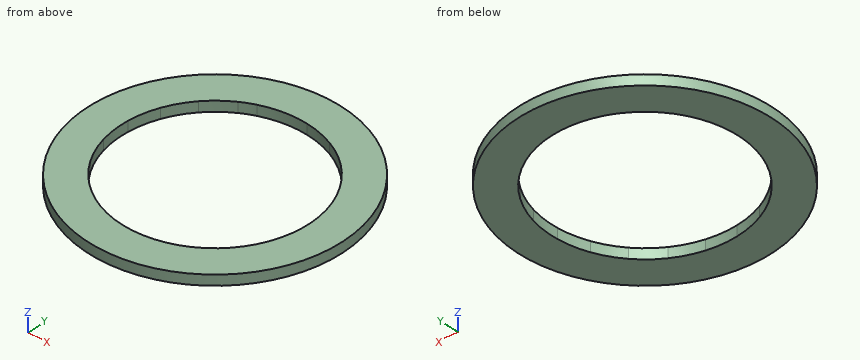
```python
from build123d import *

# Parameters (mm, degrees)
ESQUISSE1_R                  = 20
ESQUISSE1_R_2                = 16.385
BASE_EXTRUSION_DEPTH         = 1.6
BOSS_EXTRU_5_DEPTH           = 1.6
R_P_TITION_CIRCULAIRE2_COUNT = 20


with BuildPart() as part:
    # Esquisse1 → Base-Extrusion (new body)
    with BuildSketch(Plane.XY):
        Circle(ESQUISSE1_R)
        Circle(ESQUISSE1_R_2, mode=Mode.SUBTRACT)
    extrude(amount=BASE_EXTRUSION_DEPTH)

    # Esquisse3 → Boss.-Extru.5 (add)
    with BuildSketch(Plane.XY.offset(1.6)):
        with BuildLine():
            Line((1.628948568, 15.499589628), (1.398577628, 14.834398125))
            Line((1.398577628, 14.834398125), (1.195374634, 14.690915144))
            ThreePointArc((1.195374634, 14.690915144), (-2.305760746, 14.558000401), (-5.676611278, 13.602499501))
            Line((-5.676611278, 13.602499501), (-5.914207488, 13.676166747))
            Line((-5.914207488, 13.676166747), (-6.338858752, 14.237612925))
            ThreePointArc((-6.338858752, 14.237612925), (-6.917683544, 14.610159172), (-7.600152086, 14.520350848))
            ThreePointArc((-7.600152086, 14.520350848), (-2.563821531, 16.187332073), (2.74113899, 16.158250448))
            ThreePointArc((2.74113899, 16.158250448), (2.064320537, 16.032768861), (1.628948568, 15.499589628))
        make_face()
    boss_extru_5 = extrude(amount=-BOSS_EXTRU_5_DEPTH)

    # Répétition circulaire2: Boss.-Extru.5 ×20 about axis
    r_p_tition_circulaire2_axis = Axis((0, 0, 0), (0, 0, -1))
    for i in range(1, R_P_TITION_CIRCULAIRE2_COUNT):
        add(boss_extru_5.rotate(r_p_tition_circulaire2_axis, i * 360 / R_P_TITION_CIRCULAIRE2_COUNT))


solid = part.part
```
Work out the finished part from the listing and answer in its coordinate system (mm). Round coordinates to 2 decimals unless told otherwise and drop trailing zeros. Order: outer loops, then holes, each group sorted by start corner. A loop starts at its lowest first (then second) coordinate and runs counter-clockwise, first axis right, second up.
Q1. Find the intervals of material crossed by line 1 along X through (y, z) = (-1.5, 0.7); line 2 along Y through (x, z) = (-12, 0.3); line 3 along Y through (x, z) = (-5, 1.35), in increasing order.
Solution:
line 1: x = -19.94 to -14.66, 14.66 to 19.94
line 2: y = -16 to -8.56, 8.56 to 16
line 3: y = -19.36 to -13.87, 13.87 to 19.36
Q2. A cutting plane is placed at A-A, the plane y = 0. Determine the outline of the cut face in (x, z), then the cut area to 3 significant figures.
Solution:
outline: (-20, 0) - (-14.74, 0) - (-14.74, 1.6) - (-20, 1.6) - close; (14.74, 0) - (20, 0) - (20, 1.6) - (14.74, 1.6) - close
area: 16.8 mm2
Q3. A cutting plane is placed at C-C, the plane z = 0.8. Determine the outline of the cut face in (x, y).
Solution:
outline: circle Ø40 at (0, 0); hole circle Ø29.48 at (0, 0)
